from build123d import *

# Parameters (mm, degrees)
CROQUIS1_W              = 235
CROQUIS1_H              = 185
CROQUIS1_W_2            = 177
CROQUIS1_H_2            = 133
SALIENTE_EXTRUIR1_DEPTH = 4
CROQUIS2_W              = 235
CROQUIS2_H              = 185
CROQUIS2_W_2            = 188
CROQUIS2_H_2            = 142
SALIENTE_EXTRUIR2_DEPTH = 0.8
CROQUIS3_R              = 2.125
CORTAR_EXTRUIR1_DEPTH   = 5
CROQUIS4_W              = 12
CROQUIS4_H              = 11
CORTAR_EXTRUIR2_DEPTH   = 1.2


with BuildPart() as part:
    # Croquis1 → Saliente-Extruir1 (new body)
    with BuildSketch(Plane(origin=(0, 0, 0), x_dir=(1, 0, 0), z_dir=(0, 1, 0))):
        Rectangle(CROQUIS1_W, CROQUIS1_H)
        Rectangle(CROQUIS1_W_2, CROQUIS1_H_2, mode=Mode.SUBTRACT)
    extrude(amount=SALIENTE_EXTRUIR1_DEPTH)

    # Croquis2 → Saliente-Extruir2 (add)
    with BuildSketch(Plane.XZ):
        Rectangle(CROQUIS2_W, CROQUIS2_H)
        Rectangle(CROQUIS2_W_2, CROQUIS2_H_2, mode=Mode.SUBTRACT)
    extrude(amount=SALIENTE_EXTRUIR2_DEPTH)

    # Croquis3 → Cortar-Extruir1 (cut)
    with BuildSketch(Plane(origin=(0, 4, 0), x_dir=(1, 0, 0), z_dir=(0, 1, 0))):
        with Locations(Location((-107.5, 82.5, 0), (0, 0, 270))):
            Circle(CROQUIS3_R)
        with Locations(Location((-107.5, -82.5, 0), (0, 0, 270))):
            Circle(CROQUIS3_R)
        with Locations(Location((107.5, 82.5, 0), (0, 0, 270))):
            Circle(CROQUIS3_R)
        with Locations(Location((107.5, -82.5, 0), (0, 0, 270))):
            Circle(CROQUIS3_R)
    extrude(amount=-CORTAR_EXTRUIR1_DEPTH, mode=Mode.SUBTRACT)

    # Croquis4 → Cortar-Extruir2 (cut)
    with BuildSketch(Plane.XZ.offset(0.8)):
        with Locations((-100, 5.5)):
            Rectangle(CROQUIS4_W, CROQUIS4_H)
        with Locations((-100, -5.5)):
            Rectangle(CROQUIS4_W, CROQUIS4_H)
        with Locations((100, 5.5)):
            Rectangle(CROQUIS4_W, CROQUIS4_H)
        with Locations((100, -5.5)):
            Rectangle(CROQUIS4_W, CROQUIS4_H)
    extrude(amount=-CORTAR_EXTRUIR2_DEPTH, mode=Mode.SUBTRACT)


solid = part.part
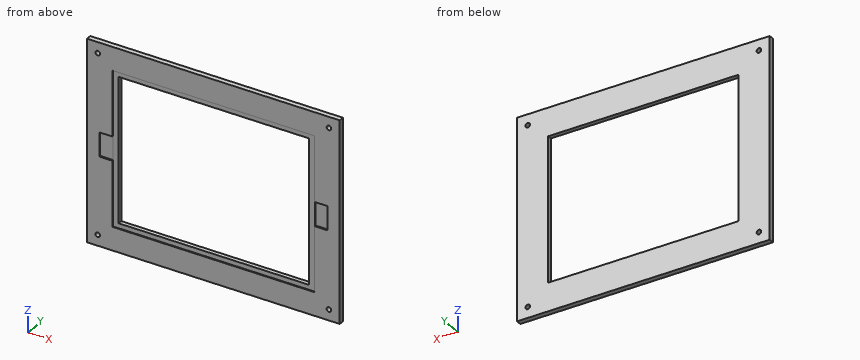
The model under review builds one solid part; all positions refer to its coordinate system, in mm. Round coordinates to 2 decimals unless told otherwise and drop trailing zeros. Loops run counter-clockwise (first coordinate to the right, second up) from the corner with the lowest first, then second, coordinate; pieces in that order, holes last. Notation, with made-up numbers: (31, 25.5) -> (53, 25.5) arc R29 cw to (53, 62.5) -> close; hole circle Ø6 at (15, 73). An arc over 180 degrees is marked (long way). One line per question, with ' | ' between items. Start each with the question number.
Item 1: Add section A-A, the plane y = 2.45. Write out the cut boundary in (x, z) (3 decimals), then the cut area to 3 significant figures.
Item 2: Add section C-C, the plane z = 32. Write out the cut boundary in (x, y).
Item 3: Wall thickness on line 1 along X through (y, z) = (2.2, 82.5) (3 decimals); line 2 along X through (y, z) = (0.8, -5.5); line 3 along Z through (x, y) = (27, -0.4): over which ranges is each line inside the solid? List them lowest first. Write a range as [from, to].
Item 4: For pin 1 (3.5 mm diameter, centred on x = 97.5, z = 0.5, fed in from -Y), flat-tipped, find the tip position at first contact; note if it passes through.
Item 5: Add section B-B, the plane x = 23.5. Write out the cut boundary in (y, z), then the cut area to 3 significant figures.
Return value:
1) outline: (-117.5, -92.5) -> (117.5, -92.5) -> (117.5, 92.5) -> (-117.5, 92.5) -> close; hole circle Ø4.25 at (-107.5, -82.5); hole circle Ø4.25 at (-107.5, 82.5); hole (-88.5, -66.5) -> (88.5, -66.5) -> (88.5, 66.5) -> (-88.5, 66.5) -> close; hole circle Ø4.25 at (107.5, -82.5); hole circle Ø4.25 at (107.5, 82.5) | area: 19,900 mm2
2) outline: (-117.5, -0.8) -> (-94, -0.8) -> (-94, 0) -> (-88.5, 0) -> (-88.5, 4) -> (-117.5, 4) -> close; (88.5, 0) -> (94, 0) -> (94, -0.8) -> (117.5, -0.8) -> (117.5, 4) -> (88.5, 4) -> close
3) line 1: x = [-117.5, -109.625], [-105.375, 105.375], [109.625, 117.5] | line 2: x = [-117.5, -88.5], [88.5, 117.5] | line 3: z = [-92.5, -71], [71, 92.5]
4) pin 1: stops at y = 0.4
5) outline: (-0.8, -92.5) -> (4, -92.5) -> (4, -66.5) -> (0, -66.5) -> (0, -71) -> (-0.8, -71) -> close; (-0.8, 71) -> (0, 71) -> (0, 66.5) -> (4, 66.5) -> (4, 92.5) -> (-0.8, 92.5) -> close | area: 242 mm2
